Verification items for the finished model (mm, model axes). A direction names the side the tool comes from. Round coordinates to 2 decimals unless told otherwise and drop trailing zeros. Order: outer loops, then holes, each group sorted by start corner. A loop starts at its lowest first (then second) coordinate and runs counter-clockwise, first axis right, second up. Notation, with made-up numbers: (71.5, 37) -> (102.5, 37) arc R15 cw to (102.5, 64) -> close; hole circle Ø10 at (15, 0.5). An arc over 180 degrees is marked (long way). Write item = value, one per line. Start each with the question number.
from build123d import *

# Parameters (mm, degrees)
EXTRUDE7_START     = 10
SKETCH1_W          = 72
SKETCH1_H          = 88
SKETCH1_R          = 14.05
SKETCH1_R_2        = 2.25
EXTRUDE7_DEPTH     = 30
SKETCH7_R          = 2.25
CUT_EXTRUDE5_DEPTH = 30


with BuildPart() as part:
    # Sketch1 → Extrude7 (new body)
    with BuildSketch(Plane.XY.offset(EXTRUDE7_START)):
        with Locations((-16, 0)):
            Rectangle(SKETCH1_W, SKETCH1_H)
        Circle(SKETCH1_R, mode=Mode.SUBTRACT)
        with Locations((-13.435028843, 13.435028843)):
            Circle(SKETCH1_R_2, mode=Mode.SUBTRACT)
        with Locations((0, 19)):
            Circle(SKETCH1_R_2, mode=Mode.SUBTRACT)
        with Locations((13.435028843, 13.435028843)):
            Circle(SKETCH1_R_2, mode=Mode.SUBTRACT)
        with Locations((13.435028843, -13.435028843)):
            Circle(SKETCH1_R_2, mode=Mode.SUBTRACT)
        with Locations((0, -19)):
            Circle(SKETCH1_R_2, mode=Mode.SUBTRACT)
        with Locations((-13.435028843, -13.435028843)):
            Circle(SKETCH1_R_2, mode=Mode.SUBTRACT)
    extrude(amount=EXTRUDE7_DEPTH)

    # Sketch7 → Cut-Extrude5 (cut)
    with BuildSketch(Plane.ZY.offset(52)):
        with Locations((17.5, 39)):
            Circle(SKETCH7_R)
        with Locations((17.5, 19)):
            Circle(SKETCH7_R)
        with Locations((17.5, -39)):
            Circle(SKETCH7_R)
        with Locations((17.5, -19)):
            Circle(SKETCH7_R)
        with Locations((17.5, 0)):
            Circle(SKETCH7_R)
        with Locations((32.5, -39)):
            Circle(SKETCH7_R)
        with Locations((32.5, -19)):
            Circle(SKETCH7_R)
        with Locations((32.5, 0)):
            Circle(SKETCH7_R)
        with Locations((32.5, 19)):
            Circle(SKETCH7_R)
        with Locations((32.5, 39)):
            Circle(SKETCH7_R)
    extrude(amount=-CUT_EXTRUDE5_DEPTH, mode=Mode.SUBTRACT)


solid = part.part
(1) Depth check by flat-ended pin: pin 1 (3.5 mm diameter, centred on y = 39, z = 17.5, fed in from -X). Enter the tip coordinate at first touch or a pass-through.
(2) Scan lines: line 1 along Y through (x, z) = (-29.75, 32.5); line 2 along Z through (x, y) = (-33, 37.5); line 3 along Y through (x, z) = (2, 29.75). Record each from-to range of solid material in increasing order. Write a range as from..to.
(3) Draft check along Z on faces 3 (the cylindrical face through (-0.488, -21.196, 24.79)), 4 (the flat face through (-22, 19, 32)), 5 (the flat face through (-17, 1, 40)). Enter one of: +Z half, -Z half, draft (parallel to the pull), parting line (faces both ways), or undercut.
(4) Cross-section at B-B (x = -47). Give the number of separate pieces and of enclosed holes in the cut face, and give its area (3 significant figures).
(5) Set-up check for faces 1 (the flat face through (20, -1, 25)), 2 (the flat face through (-22, 39, 17)): record each of +Z, -Z, +X, -X, +Y, -Y from which the full face is reachable in a straight line by a thin tool's end or side.
(6) Cross-section at D-D (y = 0). Enter the section's corners in (x, z), and give its area (3 significant figures).
(7) Cross-section at A-A (y = 19). Enter the section's corners in (x, z).
Outcome:
q1.pin_1 = -22
q2.line_1 = -44..-41.25, -36.75..-21.25, -16.75..-2.25, 2.25..16.75, 21.25..36.75, 41.25..44
q2.line_2 = 10..15.82, 19.18..30.82, 34.18..40
q2.line_3 = -44..-20.03, -17.97..-13.91, 13.91..17.97, 20.03..44
q3.face_3 = draft
q3.face_4 = undercut
q3.face_5 = +Z half
q4.separate_pieces = 1
q4.enclosed_holes = 10
q4.area = 2,480 mm^2
q5.face_1 = +Z, -Z, +X, +Y, -Y
q5.face_2 = -X
q6.outline = (-52, 10) -> (-14.05, 10) -> (-14.05, 40) -> (-52, 40) -> (-52, 34.75) -> (-22, 34.75) -> (-22, 30.25) -> (-52, 30.25) -> (-52, 19.75) -> (-22, 19.75) -> (-22, 15.25) -> (-52, 15.25) -> close; (14.05, 10) -> (20, 10) -> (20, 40) -> (14.05, 40) -> close
q6.area = 1,050 mm^2
q7.outline = (-52, 10) -> (-2.25, 10) -> (-2.25, 40) -> (-52, 40) -> (-52, 34.75) -> (-22, 34.75) -> (-22, 30.25) -> (-52, 30.25) -> (-52, 19.75) -> (-22, 19.75) -> (-22, 15.25) -> (-52, 15.25) -> close; (2.25, 10) -> (20, 10) -> (20, 40) -> (2.25, 40) -> close
